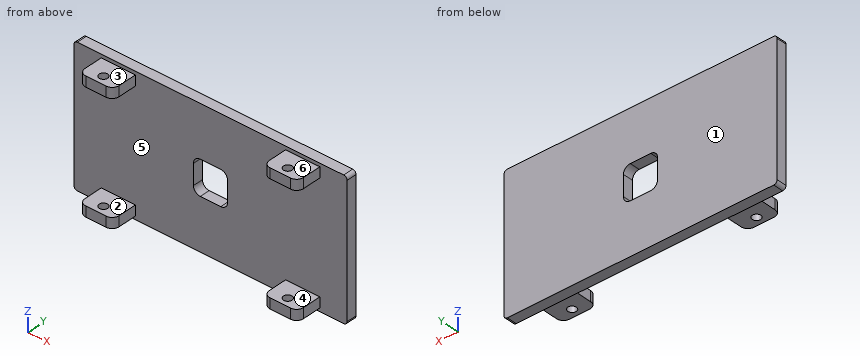
```python
from build123d import *

# Parameters (mm, degrees)
SKETCH1_W           = 800
SKETCH1_H           = 400
BOSS_EXTRUDE1_DEPTH = 30
SKETCH3_W           = 100
SKETCH3_H           = 100
CUT_EXTRUDE1_DEPTH  = 895.930164873
FILLET1_R           = 20
SKETCH4_W           = 100
SKETCH4_H           = 30
BOSS_EXTRUDE2_DEPTH = 75
SKETCH5_R           = 12.5
CUT_EXTRUDE2_DEPTH  = 894.154521905
SKETCH6_R           = 12.5
CUT_EXTRUDE3_DEPTH  = 894.154521905
FILLET2_R           = 20
FILLET3_R           = 10


with BuildPart() as part:
    # Sketch1 → Boss-Extrude1 (new body)
    with BuildSketch(Plane(origin=(0, 0, 0), x_dir=(1, 0, 0), z_dir=(0, 1, 0))):
        with Locations((400, 200)):
            Rectangle(SKETCH1_W, SKETCH1_H)
    extrude(amount=BOSS_EXTRUDE1_DEPTH)

    # Sketch3 → Cut-Extrude1 (cut, through all)
    with BuildSketch(Plane(origin=(0, 30, 0), x_dir=(1, 0, 0), z_dir=(0, 1, 0))):
        with Locations((400, 200)):
            Rectangle(SKETCH3_W, SKETCH3_H)
    extrude(amount=-CUT_EXTRUDE1_DEPTH, mode=Mode.SUBTRACT)

    # Fillet1
    fillet1_edges = [part.edges().sort_by_distance(p)[0] for p in [
        (350, 15, -250),
        (450, 15, -250),
        (450, 15, -150),
        (350, 15, -150),
    ]]
    fillet(fillet1_edges, radius=FILLET1_R)

    # Sketch4 → Boss-Extrude2 (add)
    with BuildSketch(Plane.XZ):
        with Locations((130, -25)):
            Rectangle(SKETCH4_W, SKETCH4_H)
        with Locations((670, -25)):
            Rectangle(SKETCH4_W, SKETCH4_H)
        with Locations((670, -375)):
            Rectangle(SKETCH4_W, SKETCH4_H)
        with Locations((130, -375)):
            Rectangle(SKETCH4_W, SKETCH4_H)
    extrude(amount=BOSS_EXTRUDE2_DEPTH)

    # Sketch5 → Cut-Extrude2 (cut, through all)
    with BuildSketch(Plane.XY.offset(-10)):
        with Locations((130, -50)):
            Circle(SKETCH5_R)
    extrude(amount=-CUT_EXTRUDE2_DEPTH, mode=Mode.SUBTRACT)

    # Sketch6 → Cut-Extrude3 (cut, through all)
    with BuildSketch(Plane.XY.offset(-10)):
        with Locations((670, -50)):
            Circle(SKETCH6_R)
    extrude(amount=-CUT_EXTRUDE3_DEPTH, mode=Mode.SUBTRACT)

    # Fillet2
    fillet2_edges = [part.edges().sort_by_distance(p)[0] for p in [
        (180, -75, -375),
        (80, -75, -375),
        (720, -75, -375),
        (620, -75, -375),
        (620, -75, -25),
        (720, -75, -25),
        (80, -75, -25),
        (180, -75, -25),
    ]]
    fillet(fillet2_edges, radius=FILLET2_R)

    # Fillet3
    fillet3_edges = [part.edges().sort_by_distance(p)[0] for p in [
        (0, 15, -400),
        (800, 15, -400),
        (800, 15, 0),
        (0, 15, 0),
    ]]
    fillet(fillet3_edges, radius=FILLET3_R)


solid = part.part
```
For this review, take the finished solid that the model builds, in its own axes (mm). Face numbers are marked on the shaded views. A direction names the side the tool comes from. Give positions to 0.01 mm unless a question says otherwise; leave off trailing zeros. Write each loop counter-clockwise with the first axis right and the second up, starting at its lowest first coordinate (ties: lowest second). Pieces come first, ordered by that corner, then holes. Notation, with made-up numbers: M 64,-37 L 111,-37 A11 cw 111,-23 Z; hole C 46.5,-19 d6. An arc over 180 degrees is marked long. Answer as CSV lines item,"result".
1. Draft analysis for pull direction Z (two halves, no side actions). For the marked faces 1, 2, 3 and 4, state which applies: +Z half, -Z half, draft (parallel to the pull), parting line (faces both ways), or undercut.
Findings:
face 1,"draft"
face 2,"undercut"
face 3,"+Z half"
face 4,"undercut"
2. Consider section B-B, the plane y = -14.5. Write out the cut boundary in (x, z), then the cut area to 3 significant figures.
Findings:
outline,"M 80,-390 L 180,-390 L 180,-360 L 80,-360 Z; M 80,-40 L 180,-40 L 180,-10 L 80,-10 Z; M 620,-390 L 720,-390 L 720,-360 L 620,-360 Z; M 620,-40 L 720,-40 L 720,-10 L 620,-10 Z"
area,"12,000 mm2"
3. Consider section C-C, the plane x = 380. Write out the cut boundary in (y, z).
Findings:
outline,"M 0,-400 L 30,-400 L 30,-250 L 0,-250 Z; M 0,-150 L 30,-150 L 30,0 L 0,0 Z"
4. For the marked faces 5 and 6, list the 3-axis set-ups (+Z, -Z, +X, -X, +Y, -Y) from which the entire face can be reached by the end or side of a thin tool; tool diameter is ignored.
Findings:
face 5,"-Y"
face 6,"+Z, +X, -X, -Y"
5. Consider section A-A, the plane x = 130. Write out the cut boundary in (y, z), then the cut area to 3 significant figures.
Findings:
outline,"M -75,-390 L -62.5,-390 L -62.5,-360 L -75,-360 Z; M -75,-40 L -62.5,-40 L -62.5,-10 L -75,-10 Z; M -37.5,-390 L 0,-390 L 0,-400 L 30,-400 L 30,0 L 0,0 L 0,-10 L -37.5,-10 L -37.5,-40 L 0,-40 L 0,-360 L -37.5,-360 Z"
area,"15,000 mm2"
6. For pin 1 (6 mm diameter, centred on x = 375, z = -259.5, fed in from -Y); pin 2 (9 mm diameter, centred on y = -26, z = -381.5, fed in from -X); pin 3 (22.5 mm diameter, centred on x = 108.5, y = -56, fed in from -Z), all flat-tipped, find the tip position at first contact; note any pin that passes through.
Findings:
pin 1,"stops at y = 0"
pin 2,"stops at x = 80"
pin 3,"stops at z = -390"
7. Wall thickness on line 1 (Y direction, x = 130, z = -371.75); line 2 (Z direction, x = 642.5, y = -21.5); line 3 (Y direction, x = 94, z = -317.5): over which ranges is each line inside the solid? List them lowest first.
Findings:
line 1,"y = -75 to -62.5, -37.5 to 30"
line 2,"z = -390 to -360, -40 to -10"
line 3,"y = 0 to 30"
8. Consider section D-D, the plane y = 22. Write out the cut boundary in (x, z).
Findings:
outline,"M 0,-390 A10 ccw 10,-400 L 790,-400 A10 ccw 800,-390 L 800,-10 A10 ccw 790,0 L 10,0 A10 ccw 0,-10 Z; hole M 350,-230 A20 ccw 370,-250 L 430,-250 A20 ccw 450,-230 L 450,-170 A20 ccw 430,-150 L 370,-150 A20 ccw 350,-170 Z"
